from build123d import *

# Parameters (mm, degrees)
BOSS_EXTRUDE1_DEPTH = 685.8


with BuildPart() as part:
    # Sketch1 → Boss-Extrude1 (new body)
    with BuildSketch(Plane(origin=(0, 0, 0), x_dir=(0, 0, -1), z_dir=(1, 0, 0))):
        with BuildLine():
            Line((-112.268, 0), (-190.5, 0))
            Line((-190.5, 0), (-190.5, 121.92))
            Line((-190.5, 121.92), (-112.268, 121.92))
            Line((-112.268, 121.92), (-76.2, 121.92))
            Line((-76.2, 121.92), (-76.2, 248.92))
            Line((-76.2, 248.92), (-76.2, 350.52))
            Line((-76.2, 350.52), (-132.08, 350.52))
            Line((-132.08, 350.52), (-132.08, 223.266))
            Line((-132.08, 223.266), (-289.56, 223.266))
            Line((-289.56, 223.266), (-289.56, 350.52))
            Line((-289.56, 350.52), (-303.53, 350.52))
            ThreePointArc((-303.53, 350.52), (-376.632349663, 344.135209485), (-305.743714359, 363.096234269))
            Line((-305.743714359, 363.096234269), (-289.56, 363.096234269))
            Line((-289.56, 363.096234269), (-289.56, 454.66))
            Line((-289.56, 454.66), (-132.08, 454.66))
            Line((-132.08, 454.66), (-132.08, 363.096234269))
            Line((-132.08, 363.096234269), (-55.678443819, 363.096234269))
            ThreePointArc((-55.678443819, 363.096234269), (-129.420723475, 474.502308473), (-65.500488548, 591.82))
            Line((-65.500488548, 591.82), (-187.579, 591.82))
            Line((-187.579, 591.82), (-286.645657648, 489.751322423))
            Line((-286.645657648, 489.751322423), (-359.551855918, 560.513220743))
            Line((-359.551855918, 560.513220743), (-260.485198269, 662.58189832))
            Line((-260.485198269, 662.58189832), (-211.832451768, 615.360114952))
            Line((-211.832451768, 615.360114952), (-187.579, 615.360114952))
            Line((-187.579, 615.360114952), (-187.579, 777.24))
            Line((-187.579, 777.24), (187.579, 777.24))
            Line((187.579, 777.24), (187.579, 591.82))
            Line((187.579, 591.82), (65.500488548, 591.82))
            ThreePointArc((65.500488548, 591.82), (129.420723475, 474.502308473), (55.678443819, 363.096234269))
            Line((55.678443819, 363.096234269), (142.24, 363.096234269))
            Line((142.24, 363.096234269), (142.24, 505.46))
            Line((142.24, 505.46), (281.94, 505.46))
            Line((281.94, 505.46), (281.94, 363.096234269))
            Line((281.94, 363.096234269), (298.123714359, 363.096234269))
            ThreePointArc((298.123714359, 363.096234269), (369.012349663, 344.135209485), (295.91, 350.52))
            Line((295.91, 350.52), (281.94, 350.52))
            Line((281.94, 350.52), (281.94, 218.44))
            Line((281.94, 218.44), (142.24, 218.44))
            Line((142.24, 218.44), (142.24, 350.52))
            Line((142.24, 350.52), (63.5, 350.52))
            Line((63.5, 350.52), (63.5, 248.92))
            Line((63.5, 248.92), (134.62, 248.92))
            Line((134.62, 248.92), (134.62, 121.92))
            Line((134.62, 121.92), (210.82, 121.92))
            Line((210.82, 121.92), (210.82, 0))
            Line((210.82, 0), (134.62, 0))
            Line((134.62, 0), (134.62, 113.239883031))
            Line((134.62, 113.239883031), (76.2, 113.239883031))
            Line((76.2, 113.239883031), (76.2, 0))
            Line((76.2, 0), (-76.2, 0))
            Line((-76.2, 0), (-76.2, 113.239883031))
            Line((-76.2, 113.239883031), (-112.268, 113.239883031))
            Line((-112.268, 113.239883031), (-112.268, 0))
        make_face()
    extrude(amount=BOSS_EXTRUDE1_DEPTH)


solid = part.part
Part model, mm, in its own coordinate system. A direction names the side the tool comes from. Give positions to 0.01 mm unless a question says otherwise; leave off trailing zeros. Write each loop counter-clockwise with the first axis right and the second up, starting at its lowest first coordinate (ties: lowest second). Pieces come first, ordered by that corner, then holes.
1) Cut at D-D on z = 340.36. Write the cut outline in (x, y), then the cut area to 3 significant figures.
Resolved:
outline: (0, 313.69) - (685.8, 313.69) - (685.8, 387.35) - (0, 387.35) - close; (0, 541.89) - (685.8, 541.89) - (685.8, 580.29) - (0, 580.29) - close
area: 76,900 mm2
2) Probe L1, parallel to Z at x = 456, y = 57.5; L2, parallel to Z at x = 511, y = 271; L3, parallel to Y at x = 145, z = 170. List the from-to ranges inside material, lowest first.
Resolved:
L1: z = -210.82 to -134.62, -76.2 to 76.2, 112.27 to 190.5
L2: z = -281.94 to -142.24, -63.5 to 76.2, 132.08 to 289.56
L3: y = 0 to 121.92, 223.27 to 454.66, 591.82 to 777.24
3) Cut at B-B on y = 640. Write the cut outline in (x, z).
Resolved:
outline: (0, -187.58) - (685.8, -187.58) - (685.8, 187.58) - (0, 187.58) - close; (0, 237.22) - (685.8, 237.22) - (685.8, 282.4) - (0, 282.4) - close
4) Which spindle directions (+Z, -Z, +X, -X, +Y, -Y) get a long thin tool onto all of the face, cutting with end or side? Do faces 5 (the face through (338, 57, 112.268)), 6 (the face through (338, 121.92, -172)), 7 (the face through (338, 223.266, 210)), 8 (the face through (338, 350.52, 104)). Say none if no direction does.
Resolved:
face 5: +X, -X, -Y
face 6: -Z, +X, -X
face 7: +Z, +X, -X
face 8: +X, -X
5) Cut at A-A on z = 166.5. Write the cut outline in (x, y).
Resolved:
outline: (0, 0) - (685.8, 0) - (685.8, 121.92) - (0, 121.92) - close; (0, 223.27) - (685.8, 223.27) - (685.8, 454.66) - (0, 454.66) - close; (0, 591.82) - (685.8, 591.82) - (685.8, 777.24) - (0, 777.24) - close
6) Two-plate mould, pull along Z, no slides. Class faces 1 (the face through (338, 505.46, -211)), 2 (the face through (338, 288, 132.08)), 3 (the face through (338, 56, 76.2)), 4 (the face through (338.1, 524.64, 322.59)): released by +Z, released by -Z, zero draft, split by the parting line, or undercut.
Resolved:
face 1: zero draft
face 2: undercut
face 3: undercut
face 4: released by +Z
7) Cut at C-C on z = -94. Write the cut outline in (x, y).
Resolved:
outline: (0, 113.24) - (685.8, 113.24) - (685.8, 248.92) - (0, 248.92) - close; (0, 350.52) - (685.8, 350.52) - (685.8, 363.1) - (0, 363.1) - close; (0, 390.93) - (685.8, 390.93) - (685.8, 569.19) - (0, 569.19) - close; (0, 591.82) - (685.8, 591.82) - (685.8, 777.24) - (0, 777.24) - close
8) Pin check, flat tips, straight feed: pin 1 (4 mm diameter, centred on x = 427.5, z = 294, fed in from -Y); pin 2 (10 mm diameter, centred on x = 198.5, y = 335, fed in from +Z); pin 3 (7.5 mm diameter, centred on x = 442.5, z = 198, fed in from +Y). Stop position of each tip, or through.
Resolved:
pin 1: stops at y = 350.52
pin 2: stops at z = 375.66
pin 3: stops at y = 615.36
